```python
from build123d import *

# Parameters (mm, degrees)
SKETCH2_W           = 69
SKETCH2_H           = 84
SKETCH2_W_2         = 65
SKETCH2_H_2         = 80
BOSS_EXTRUDE1_DEPTH = 13
SKETCH3_OUTSIDE_W   = 92.896
SKETCH3_OUTSIDE_H   = 107.896
SKETCH3_OUTSIDE_W_2 = 67
SKETCH3_OUTSIDE_H_2 = 82
CUT_EXTRUDE1_DEPTH  = 3
SKETCH4_W           = 69
SKETCH4_H           = 84
BOSS_EXTRUDE2_DEPTH = 2
FILLET1_R           = 3
CUT_EXTRUDE2_DEPTH  = 3
LPATTERN1_COUNT     = 14
LPATTERN1_PITCH     = 5
SKETCH6_R           = 4
BOSS_EXTRUDE3_DEPTH = 10
CUT_EXTRUDE3_REACH  = 58.385
SKETCH7_R           = 3
FILLET2_R           = 2
BOSS_EXTRUDE4_START = -2
SKETCH8_R           = 4
SKETCH8_R_2         = 1.5
BOSS_EXTRUDE4_DEPTH = 2
SKETCH10_W          = 2
SKETCH10_H          = 7
CUT_EXTRUDE4_DEPTH  = 3
FILLET10_R          = 1


with BuildPart() as part:
    # Sketch2 → Boss-Extrude1 (new body)
    with BuildSketch(Plane.XY):
        Rectangle(SKETCH2_W, SKETCH2_H)
        Rectangle(SKETCH2_W_2, SKETCH2_H_2, mode=Mode.SUBTRACT)
    extrude(amount=BOSS_EXTRUDE1_DEPTH)

    # Sketch3 outside → Cut-Extrude1 (cut)
    with BuildSketch(Plane.XY.offset(13)):
        Rectangle(SKETCH3_OUTSIDE_W, SKETCH3_OUTSIDE_H)
        Rectangle(SKETCH3_OUTSIDE_W_2, SKETCH3_OUTSIDE_H_2, mode=Mode.SUBTRACT)
    extrude(amount=-CUT_EXTRUDE1_DEPTH, mode=Mode.SUBTRACT)

    # Sketch4 → Boss-Extrude2 (add)
    with BuildSketch(Plane(origin=(0, 0, 0), x_dir=(-1, 0, 0), z_dir=(0, 0, -1))):
        Rectangle(SKETCH4_W, SKETCH4_H)
    extrude(amount=BOSS_EXTRUDE2_DEPTH)

    # Fillet1
    fillet1_edges = [part.edges().sort_by_distance(p)[0] for p in [
        (32.5, -40, 6.5),
        (32.5, 40, 6.5),
        (-32.5, 40, 6.5),
        (-32.5, -40, 6.5),
        (34.5, -42, 4),
        (-34.5, -42, 4),
        (-34.5, 42, 4),
        (34.5, 42, 4),
        (33.5, -41, 11.5),
        (-33.5, -41, 11.5),
        (-33.5, 41, 11.5),
        (33.5, 41, 11.5),
    ]]
    fillet(fillet1_edges, radius=FILLET1_R)

    # Sketch5 → Cut-Extrude2 (cut)
    with BuildSketch(Plane(origin=(34.5, 0, 0), x_dir=(0, 0, -1), z_dir=(1, 0, 0))):
        with BuildLine():
            Line((-4, -33), (-13, -33))
            Line((-13, -33), (-13, -31))
            Line((-13, -31), (-4, -31))
            ThreePointArc((-4, -31), (-3, -32), (-4, -33))
        make_face()
    cut_extrude2 = extrude(amount=-CUT_EXTRUDE2_DEPTH, mode=Mode.SUBTRACT)

    # LPattern1: Cut-Extrude2 ×14
    with Locations(*[(0, i * LPATTERN1_PITCH, 0) for i in range(1, LPATTERN1_COUNT)]):
        add(cut_extrude2, mode=Mode.SUBTRACT)

    # Sketch6 → Boss-Extrude3 (add)
    with BuildSketch(Plane.XY):
        with Locations(Location((27.5, 35, 0), (0, 0, 180))):
            Circle(SKETCH6_R)
        with Locations(Location((-27.5, -35, 0), (0, 0, 180))):
            Circle(SKETCH6_R)
    extrude(amount=BOSS_EXTRUDE3_DEPTH)

    # Sketch7 → Cut-Extrude3 (cut, up to next)
    with BuildSketch(Plane(origin=(0, 0, -2), x_dir=(-1, 0, 0), z_dir=(0, 0, -1)), mode=Mode.PRIVATE) as cut_extrude3_sk1:
        with Locations((27.5, -35)):
            Circle(SKETCH7_R)
    cut_extrude3_tool1 = extrude(cut_extrude3_sk1.sketch, amount=-CUT_EXTRUDE3_REACH, mode=Mode.PRIVATE) & part.part
    # Sketch7 → Cut-Extrude3 (cut, up to next)
    with BuildSketch(Plane(origin=(0, 0, -2), x_dir=(-1, 0, 0), z_dir=(0, 0, -1)), mode=Mode.PRIVATE) as cut_extrude3_sk2:
        with Locations((-27.5, 35)):
            Circle(SKETCH7_R)
    cut_extrude3_tool2 = extrude(cut_extrude3_sk2.sketch, amount=-CUT_EXTRUDE3_REACH, mode=Mode.PRIVATE) & part.part
    add(cut_extrude3_tool1.solids().sort_by_distance((-27.5, -35, -2))[0], mode=Mode.SUBTRACT)
    add(cut_extrude3_tool2.solids().sort_by_distance((27.5, 35, -2))[0], mode=Mode.SUBTRACT)

    # Fillet2
    fillet2_edges = [part.edges().sort_by_distance(p)[0] for p in [
        (-24.5, -35, -2),
        (30.5, 35, -2),
    ]]
    fillet(fillet2_edges, radius=FILLET2_R)

    # Sketch8 → Boss-Extrude4 (add)
    # profile 1 of 2: a face of its own
    with BuildSketch(Plane.XY.offset(10).offset(BOSS_EXTRUDE4_START)):
        with Locations(Location((-27.5, -35, 0), (0, 0, 180))):
            Circle(SKETCH8_R)
        with Locations((-27.5, -35)):
            Circle(SKETCH8_R_2, mode=Mode.SUBTRACT)
    # profile 2 of 2: a face of its own
    with BuildSketch(Plane.XY.offset(10).offset(BOSS_EXTRUDE4_START)):
        with Locations(Location((27.5, 35, 0), (0, 0, 180))):
            Circle(SKETCH8_R)
        with Locations((27.5, 35)):
            Circle(SKETCH8_R_2, mode=Mode.SUBTRACT)
    extrude(amount=BOSS_EXTRUDE4_DEPTH)

    # Sketch10 → Cut-Extrude4 (cut)
    with BuildSketch(Plane.ZY.offset(34.5)):
        with Locations((2, 19.01524614)):
            Rectangle(SKETCH10_W, SKETCH10_H)
    extrude(amount=-CUT_EXTRUDE4_DEPTH, mode=Mode.SUBTRACT)

    # Fillet10
    fillet10_edges = [part.edges().sort_by_distance(p)[0] for p in [
        (-32.5, 22.51524614, 2),
        (-32.5, 19.01524614, 1),
        (-32.5, 15.51524614, 2),
        (-32.5, 19.01524614, 3),
    ]]
    fillet(fillet10_edges, radius=FILLET10_R - 0.0001)  # a hair under: the kernel refuses the full size


solid = part.part
```
Design review of the part built by this model. Coordinates are the model's own, in mm. A direction names the side the tool comes from. Give positions to 0.01 mm unless a question says otherwise; leave off trailing zeros. Loops run counter-clockwise (first coordinate to the right, second up) from the corner with the lowest first, then second, coordinate; pieces in that order, holes last. Notation, with made-up numbers: (8, 74.5) -> (15, 74.5) arc R30 ccw to (15, 112.5) -> close; hole circle Ø10 at (-8, 20). An arc over 180 degrees is marked (long way). One line per item, written item: value.
Q1. We need section C-C on z = 6.5. Give the number of separate pieces and of enclosed holes in the cut face, and give its area (3 significant figures).
Numbers:
separate pieces: 16
enclosed holes: 2
area: 584 mm^2
Q2. We need section B-B on x = -27.5. Give the boundary of the cut face in (y, z).
Numbers:
outline: (-42, -2) -> (-40, -2) arc R2 ccw to (-38, 0) -> (-38, 8) -> (-36.5, 8) -> (-36.5, 10) -> (-39, 10) -> (-39, 0) -> (-40, 0) -> (-40, 13) -> (-41, 13) -> (-41, 10) -> (-42, 10) -> close; (-33.5, 8) -> (-32, 8) -> (-32, 0) arc R2 ccw to (-30, -2) -> (42, -2) -> (42, 10) -> (41, 10) -> (41, 13) -> (40, 13) -> (40, 0) -> (-31, 0) -> (-31, 10) -> (-33.5, 10) -> close
Q3. We need section A-A on y = 35. Give the boundary of the cut face in (x, z).
Numbers:
outline: (-34.5, -2) -> (22.5, -2) arc R2 ccw to (24.5, 0) -> (24.5, 8) -> (26, 8) -> (26, 10) -> (23.5, 10) -> (23.5, 0) -> (-32.5, 0) -> (-32.5, 13) -> (-33.5, 13) -> (-33.5, 10) -> (-34.5, 10) -> close; (29, 8) -> (30.5, 8) -> (30.5, 0) arc R2 ccw to (32.5, -2) -> (34.5, -2) -> (34.5, 10) -> (33.5, 10) -> (33.5, 13) -> (32.5, 13) -> (32.5, 0) -> (31.5, 0) -> (31.5, 10) -> (29, 10) -> close
Q4. For pin 1 Ø2 at (x, z) = (33, 8) entering from -Y; pin 2 Ø6 at (x, y) = (-9, 8) entering from +Z; pin 3 Ø1.5 at (y, z) = (-19, 11) entering from +X, all flat-tipped, find the tip position at first contact; note any pin that passes through.
Numbers:
pin 1: stops at y = -41.96
pin 2: stops at z = 0
pin 3: stops at x = 33.5
Q5. Machinability: for faces 1 (the flat face through (33.5, -20, 12)), 2 (the flat face through (-29.2, -35.1, 10)), 3 (the flat face through (34, -13, 7)), which of the approach directions +Z, -Z, +X, -X, +Y, -Y give a long, thin tool a straight path to every point of the face, cutting with its end or side? Answer none if there is none.
Numbers:
face 1: +Z, +X, +Y, -Y
face 2: +Z
face 3: +Z, +X
Q6. For L1, parallel to Y at x = 27.5, z = 8.75; L2, parallel to X at y = 24, z = 2.25; L3, parallel to Y at x = 13, z = 5.5, list the stretches that pass through material, from the lowest coordinate up.
Numbers:
L1: y = -42 to -40, 31 to 33.5, 36.5 to 39, 40 to 42
L2: x = -34.5 to -32.5, 32.5 to 34.5
L3: y = -42 to -40, 40 to 42
Q7. We need section D-D on y = -10. Give the boundary of the cut face in (x, z), and give its area (3 significant figures).
Numbers:
outline: (-34.5, -2) -> (34.5, -2) -> (34.5, 10) -> (33.5, 10) -> (33.5, 13) -> (32.5, 13) -> (32.5, 0) -> (-32.5, 0) -> (-32.5, 13) -> (-33.5, 13) -> (-33.5, 10) -> (-34.5, 10) -> close
area: 184 mm^2
